Can you work these out from the drawing? Everything is in mm from the part's minimum corner. A direction names the side the tool comes from. Round coordinates to 2 decimals unless told otherwise and drop trailing zeros. Order: outer loops, then holes, each group sorted by start corner. A loop starts at its lowest first (then second) coordinate and runs counter-clockwise, first axis right, second up. Notation, with made-up numbers: (-27, 23.25) -> (-8, 23.25) arc R18 ccw to (-8, 46.25) -> close; hole circle Ø10 at (14, 21.5). An arc over 180 degrees is marked (long way). One line per item, written item: value.
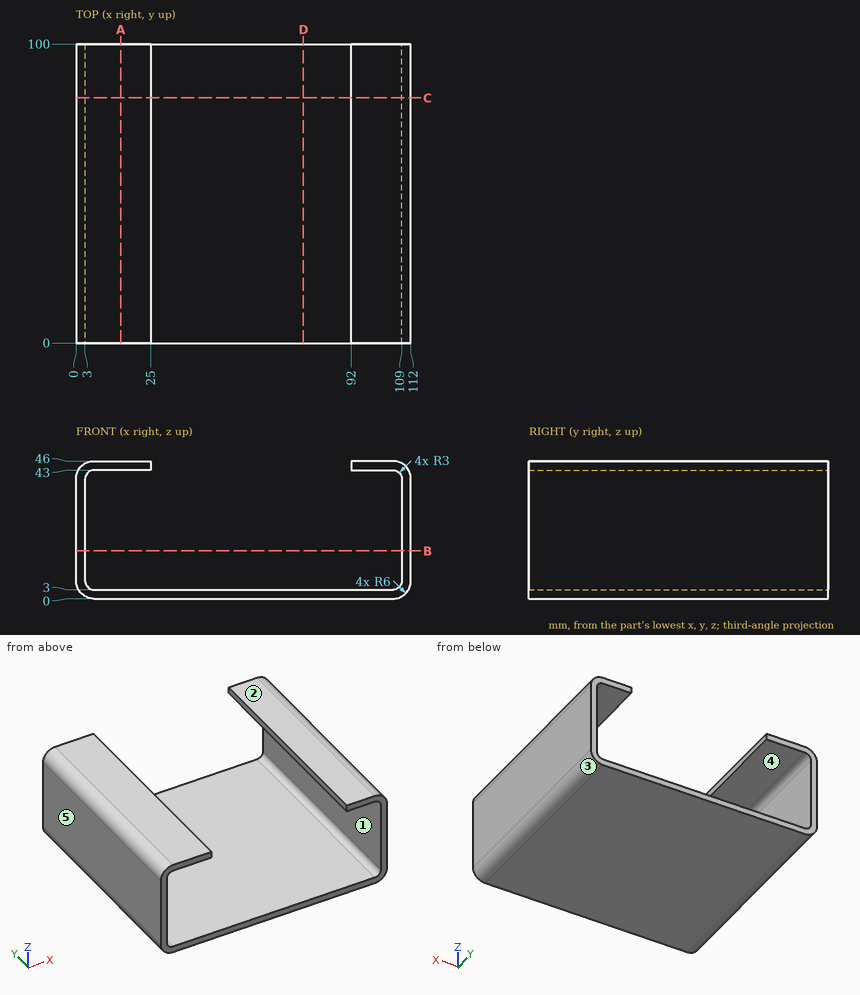
Q1. I want a section at D-D on x = 76. List the corners of the cut face in (y, z) for me.
Answers below:
outline: (0, 0) -> (100, 0) -> (100, 3) -> (0, 3) -> close
Q2. We'd pull the mould along Z, two halves only. Please class the marked faces 1, 2 and 3: released by +Z, released by -Z, zero draft, split by the parting line, or undercut.
Answers below:
face 1: undercut
face 2: released by +Z
face 3: released by -Z
Q3. Will these pins go through, and if not, where does the flat tip stop? pin 1 Ø21 at (x, y) = (12.5, 39) entering from -Z; pin 2 Ø2.5 at (y, z) = (67.5, 45) entering from +X; pin 3 Ø1.5 at (y, z) = (50, 44) entering from -X.
Answers below:
pin 1: z = 0
pin 2: x = 110.68
pin 3: x = 0.96
Q4. On a 3-axis mill with a long thin cutter (end or side, diameter ignored), from which of +Z, -Z, +X, -X, +Y, -Y can I reach the whole of each face in a straight line? I mean the marked faces 4 and 5. Say none if no direction works.
Answers below:
face 4: +Y, -Y
face 5: +Z, -Z, -X, +Y, -Y
Q5. I want a section at C-C on y = 82. List the corners of the cut face in (x, z) for me.
Answers below:
outline: (0, 6) arc R6 ccw to (6, 0) -> (106, 0) arc R6 ccw to (112, 6) -> (112, 40) arc R6 ccw to (106, 46) -> (92, 46) -> (92, 43) -> (106, 43) arc R3 cw to (109, 40) -> (109, 6) arc R3 cw to (106, 3) -> (6, 3) arc R3 cw to (3, 6) -> (3, 40) arc R3 cw to (6, 43) -> (25, 43) -> (25, 46) -> (6, 46) arc R6 ccw to (0, 40) -> close
Q6. I want a section at B-B on z = 16. List the corners of the cut face in (x, y) for me.
Answers below:
outline: (0, 0) -> (3, 0) -> (3, 100) -> (0, 100) -> close; (109, 0) -> (112, 0) -> (112, 100) -> (109, 100) -> close
Q7. I want a section at A-A on x = 15. List the corners of the cut face in (y, z) for me, plus the area to 3 significant figures.
Answers below:
outline: (0, 0) -> (100, 0) -> (100, 3) -> (0, 3) -> close; (0, 43) -> (100, 43) -> (100, 46) -> (0, 46) -> close
area: 600 mm^2
Q8. Please list where these lines run through material, in increasing order: line 1 along Z through (x, y) = (7, 54); line 2 along X through (y, z) = (32.5, 12); line 3 along Z through (x, y) = (48, 96).
Answers below:
line 1: 0 to 3, 43 to 46
line 2: 0 to 3, 109 to 112
line 3: 0 to 3
